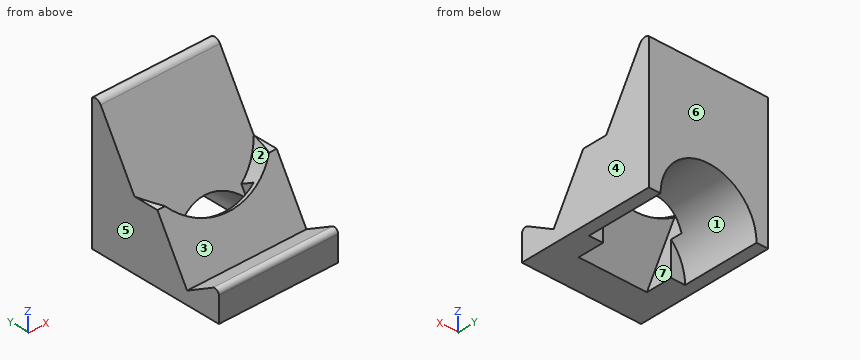
```python
from build123d import *

# Parameters (mm, degrees)
F1_DEPTH  = 88.9
F3_DEPTH  = 15.875
F5_DEPTH  = 88.901
F6_W      = 50.8
F6_H      = 11.43
F7_DEPTH  = 136.4343795657
F8_R      = 35.7660342863
F9_DEPTH  = 57.15
F10_W     = 50.8
F10_H     = 6.2183902673
F11_DEPTH = 10.7715678842
F13_DEPTH = 88.9
F15_DEPTH = 88.901
F17_DEPTH = 88.901


with BuildPart() as f1:
    # F0 (on Right) → F1 (new body)
    with BuildSketch(Plane.YZ):
        Polygon((0, 9.525), (0, 0), (101.6, 0), (101.6, 101.6), (78.5595260356, 101.6), (25.4, 9.525), align=None)
    extrude(amount=F1_DEPTH)

    # F2 (on face) → F3 (cut)
    with BuildSketch(Plane(origin=(0, 14.9255540145, -8.6172726281), x_dir=(1, 0, 0), z_dir=(0, -0.8660254038, 0.5))):
        with BuildLine():
            Line((0, 127.2679440423), (-3.7916075595, 108.4635424443))
            ThreePointArc((-3.7916075595, 108.4635424443), (44.45, 49.523891971), (92.6916075595, 108.4635424443))
            Line((92.6916075595, 108.4635424443), (88.9, 127.2679440423))
            Line((88.9, 127.2679440423), (88.9, 140.5219882727))
            Line((88.9, 140.5219882727), (0, 140.5219882727))
            Line((0, 140.5219882727), (0, 127.2679440423))
        make_face()
    extrude(amount=-F3_DEPTH, mode=Mode.SUBTRACT)

    # F4 (on face) → F5 (cut, through all)
    with BuildSketch(Plane.YZ.offset(88.9)):
        Polygon((103.9759144766, 114.3859309679), (96.8903970824, 101.6), (110.1333461889, 93.9541797685), (117.4411960521, 106.6117470256), align=None)
    extrude(amount=-F5_DEPTH, mode=Mode.SUBTRACT)

    # F6 (on face) → F7 (cut, through all)
    with BuildSketch(Plane(origin=(0, 68.2166897829, 118.1547726281), x_dir=(1, 0, 0), z_dir=(0, 0.5, 0.8660254038))):
        with Locations((44.45, 27.3945452561)):
            Rectangle(F6_W, F6_H)
    extrude(amount=-F7_DEPTH, mode=Mode.SUBTRACT)

    # F8 (on face) → F9 (cut)
    with BuildSketch(Plane(origin=(0, 101.6, 0), x_dir=(-1, 0, 0), z_dir=(0, 1, 0))):
        with Locations((-44.45, 0)):
            Circle(F8_R)
    extrude(amount=-F9_DEPTH, mode=Mode.SUBTRACT)

    # F10 (on face) → F11 (cut, through all)
    with BuildSketch(Plane(origin=(0, 0, 0), x_dir=(1, 0, 0), z_dir=(0, 0, -1))):
        with Locations((44.45, -41.3408048664)):
            Rectangle(F10_W, F10_H)
    extrude(amount=-F11_DEPTH, mode=Mode.SUBTRACT)

    # F12 (on face) → F13 (join)
    with BuildSketch(Plane.YZ.offset(88.9)):
        with BuildLine():
            Line((0, 9.525), (25.4, 9.525))
            Line((25.4, 9.525), (4.7625, 21.4400661804))
            ThreePointArc((4.7625, 21.4400661804), (1.5875, 21.4400661804), (0, 18.6904355234))
            Line((0, 18.6904355234), (0, 9.525))
        make_face()
    extrude(amount=-F13_DEPTH)

    # F14 (on face) → F15 (cut, through all)
    with BuildSketch(Plane.YZ.offset(88.9)):
        Polygon((49.1508753236, 50.6627227848), (67.4817463704, 50.6627227848), (53.7335930853, 58.6002227848), align=None)
    extrude(amount=-F15_DEPTH, mode=Mode.SUBTRACT)

    # F16 (on face) → F17 (cut, through all)
    with BuildSketch(Plane.YZ.offset(88.9)):
        with BuildLine():
            ThreePointArc((94.5091470824, 97.4755540145), (97.4009673604, 99.6945257608), (101.0148430585, 99.2187500055))
            Line((101.0148430585, 99.2187500055), (96.8903970824, 101.6))
            Line((96.8903970824, 101.6), (94.5091470824, 97.4755540145))
        make_face()
        with BuildLine():
            ThreePointArc((101.0148430585, 99.2187500055), (101.3148393446, 99.0303330608), (101.6, 98.8201376344))
            Line((101.6, 98.8201376344), (101.6, 98.8809094878))
            Line((101.6, 98.8809094878), (101.0148430585, 99.2187500055))
        make_face()
    extrude(amount=-F17_DEPTH, mode=Mode.SUBTRACT)


solid = f1.part
```
Check sheet for the modelled part. Datum: model origin and axes. Units: mm. Face numbers are marked on the shaded views. A direction names the side the tool comes from. Coordinates: 2 decimals unless noted, no trailing zeros. Loops run counter-clockwise (first coordinate to the right, second up) from the corner with the lowest first, then second, coordinate; pieces in that order, holes last.
1) Sectioned sample at B-B (z = 16). Record the boundary of the cut face in (x, y), and give its area (3 significant figures).
2) Material ranges on probe 1 along X at (y, z) = (42, 20); probe 2 along Y at (x, z) = (31, 20.5), recorded low to high.
3) Release check for a two-part mould opening along X. For the marked faces 4, 5, 6 and 7 record: released by +X, released by -X, zero draft, split by the parting line, or undercut.
4) Sectioned sample at C-C (y = 33). Record the boundary of the cut face in (x, z).
5) Access from +Z, -Z, +X, -X, +Y, -Y to the whole of each face (thin tool, end or side, straight path). Record for the marked faces 1, 2 and 3.
6) Gauge pin test, flat ends, axial feed: pin 1 (8 mm diameter, centred on x = 74.5, y = 24, fed in from +Z); pin 2 (5 mm diameter, centred on x = 40, y = 76, fed in from +Z); pin 3 (4.5 mm diameter, centred on x = 2, y = 62.5, fed in from +Z). Record the tip position at first contact, or that the pin passes through.
Check sheet entries:
1. outline: (0, 0) - (88.9, 0) - (88.9, 14.18) - (0, 14.18) - close; (0, 29.14) - (88.9, 29.14) - (88.9, 101.6) - (76.44, 101.6) - (76.44, 44.45) - (69.85, 44.45) - (69.85, 34.27) - (19.05, 34.27) - (19.05, 44.45) - (12.46, 44.45) - (12.46, 101.6) - (0, 101.6) - close
1. area: 3,530 mm2
2. probe 1: x = 0 to 19.05, 69.85 to 88.9
2. probe 2: y = 0.57 to 6.39, 31.74 to 36.87
3. face 4: released by +X
3. face 5: released by -X
3. face 6: zero draft
3. face 7: undercut
4. outline: (0, 0) - (19.05, 0) - (19.05, 13.8) - (69.85, 13.8) - (69.85, 0) - (88.9, 0) - (88.9, 22.69) - (0, 22.69) - close
5. face 1: -Z, +Y
5. face 2: +Z
5. face 3: +Z, +X, -X
6. pin 1: stops at z = 14.03
6. pin 2: stops at z = 69.75
6. pin 3: stops at z = 50.66
